Here's how the part is built. I have some questions about the finished solid (model axes, mm). A direction names the side the tool comes from. Give positions to 0.01 mm unless a question says otherwise; leave off trailing zeros. Loops run counter-clockwise (first coordinate to the right, second up) from the corner with the lowest first, then second, coordinate; pieces in that order, holes last. Notation, with made-up numbers: (27.5, 3.5) -> (33.5, 3.5) arc R10 cw to (33.5, 8.5) -> close; hole circle Ø2 at (68.25, -33). An arc over 180 degrees is marked (long way). Answer in a Markdown table with one row per item. Add a question column.
Item 1: For P1, Ø1.5, axis at y = 14, z = 6, coming from the -X side; P2, Ø5, axis at x = 5, z = -1, coming from the +Y side, each with a flat end and sliding along its axis, tell me the tip position at first contact or that it passes through.
Item 2: If we section it at C-C (y = 7.25): Write out the boundary of the cut face in (x, z), then the cut area to 3 significant figures.
Item 3: If we section it at A-A (z = 6): Write out the boundary of the cut face in (x, y).
Item 4: If I drill on line 1 (Z direction, x = 8.5, y = 20.5); line 2 (X direction, y = 8, z = 2.25); line 3 (Y direction, x = 5.5, z = -5.25), over which ranges is the centre line in solid material (lowest first)?
Item 5: We'd pull the mould along Z, two halves only. Please class faces 1 (the face through (3, 22.8, -7)), 2 (the face through (0, 11, 6.48)), 3 (the face through (0, 11, 7.98)): released by +Z, released by -Z, zero draft, split by the parting line, or undercut.
Item 6: If we section it at D-D (x = 8): Write out the boundary of the cut face in (y, z).
Item 7: If we section it at B-B (x = -8): Write out the boundary of the cut face in (y, z), then the cut area to 3 significant figures.
Item 8: Which directions (+Z, -Z, +X, -X, +Y, -Y) give clear straight access to the entire face, cutting with the end or side of a thin tool? Please do faces 4 (the face through (2, 0, 0)), 5 (the face through (13.12, 11, 0)), 6 (the face through (-12, 8.99, -5)), 7 (the face through (-6.38, -1, 0)).
```python
from build123d import *

# Parameters (mm, degrees)
SKETCH_13_W         = 26.24
SKETCH_13_H         = 15.96
SKETCH_13_W_2       = 23.24
SKETCH_13_H_2       = 12.96
EXTRUDE_1_DEPTH     = 22.8
SKETCH_13_3_W       = 26.24
SKETCH_13_3_H       = 15.96
SKETCH_13_3_W_2     = 23.24
SKETCH_13_3_H_2     = 12.96
SKETCH_13_3_W_3     = 18
SKETCH_13_3_W_4     = 1.92
EXTRUDE_2_DEPTH     = 1.5
CUT_EXTRUDE_4_DEPTH = 1.5


with BuildPart() as part:
    # 草图13 → 凸台-拉伸1 (new body)
    with BuildSketch(Plane(origin=(0, 0, 0), x_dir=(1, 0, 0), z_dir=(0, 1, 0))):
        Rectangle(SKETCH_13_W, SKETCH_13_H)
        Rectangle(SKETCH_13_W_2, SKETCH_13_H_2, mode=Mode.SUBTRACT)
    extrude(amount=EXTRUDE_1_DEPTH)

    # 草图13<3> → 凸台-拉伸2 (add)
    with BuildSketch(Plane(origin=(0, 0, 0), x_dir=(1, 0, 0), z_dir=(0, 1, 0))):
        Rectangle(SKETCH_13_3_W, SKETCH_13_3_H)
        Rectangle(SKETCH_13_3_W_2, SKETCH_13_3_H_2, mode=Mode.SUBTRACT)
        with Locations((2.62, 0)):
            Rectangle(SKETCH_13_3_W_3, SKETCH_13_3_H_2)
        with Locations((-10.66, 0)):
            Rectangle(SKETCH_13_3_W_4, SKETCH_13_3_H_2)
    extrude(amount=-EXTRUDE_2_DEPTH)

    # 草图15 → 切除-拉伸4 (cut)
    with BuildSketch(Plane.ZY.offset(13.12)):
        with BuildLine():
            ThreePointArc((-1.600781059, 8.99), (-1.015504801, 8.08951932), (0, 7.74))
            ThreePointArc((0, 7.74), (1.015504801, 8.08951932), (1.600781059, 8.99))
            Line((1.600781059, 8.99), (-1.600781059, 8.99))
        make_face()
        with BuildLine():
            ThreePointArc((1.65, 9.39), (-0.201508377, 11.027649039), (-1.600781059, 8.99))
            Line((-1.600781059, 8.99), (1.600781059, 8.99))
            ThreePointArc((1.600781059, 8.99), (1.637649039, 9.188491623), (1.65, 9.39))
        make_face()
        with BuildLine():
            Line((-7.98, 22.8), (-7.98, 8.99))
            Line((-7.98, 8.99), (-1.600781059, 8.99))
            ThreePointArc((-1.600781059, 8.99), (-0.201508377, 11.027649039), (1.65, 9.39))
            ThreePointArc((1.65, 9.39), (1.637649039, 9.188491623), (1.600781059, 8.99))
            Line((1.600781059, 8.99), (7.98, 8.99))
            Line((7.98, 8.99), (7.98, 22.8))
            Line((7.98, 22.8), (-7.98, 22.8))
        make_face()
    extrude(amount=-CUT_EXTRUDE_4_DEPTH, mode=Mode.SUBTRACT)


solid = part.part
```
Recorded:
| question | item | result |
|---|---|---|
| 1 | P1 | stops at x = -11.62 |
| 1 | P2 | stops at y = 0 |
| 2 | outline | (-13.12, -7.98) -> (13.12, -7.98) -> (13.12, 7.98) -> (-13.12, 7.98) -> close; hole (-11.62, -6.48) -> (11.62, -6.48) -> (11.62, 6.48) -> (-11.62, 6.48) -> close |
| 2 | area | 118 mm^2 |
| 3 | outline | (-13.12, -1.5) -> (-9.7, -1.5) -> (-9.7, 0) -> (-11.62, 0) -> (-11.62, 8.99) -> (-13.12, 8.99) -> close; (-6.38, -1.5) -> (13.12, -1.5) -> (13.12, 22.8) -> (11.62, 22.8) -> (11.62, 0) -> (-6.38, 0) -> close |
| 4 | line 1 | z = -7.98 to -6.48, 6.48 to 7.98 |
| 4 | line 2 | x = -13.12 to -11.62, 11.62 to 13.12 |
| 4 | line 3 | y = -1.5 to 0 |
| 5 | face 1 | zero draft |
| 5 | face 2 | undercut |
| 5 | face 3 | released by +Z |
| 6 | outline | (-1.5, -7.98) -> (22.8, -7.98) -> (22.8, -6.48) -> (0, -6.48) -> (0, 6.48) -> (22.8, 6.48) -> (22.8, 7.98) -> (-1.5, 7.98) -> close |
| 7 | outline | (-1.5, -7.98) -> (22.8, -7.98) -> (22.8, -6.48) -> (-1.5, -6.48) -> close; (-1.5, 6.48) -> (22.8, 6.48) -> (22.8, 7.98) -> (-1.5, 7.98) -> close |
| 7 | area | 72.9 mm^2 |
| 8 | face 4 | +Y |
| 8 | face 5 | +Z, -Z, +X, +Y, -Y |
| 8 | face 6 | +Z, -Z, -X, +Y |
| 8 | face 7 | +Y, -Y |
